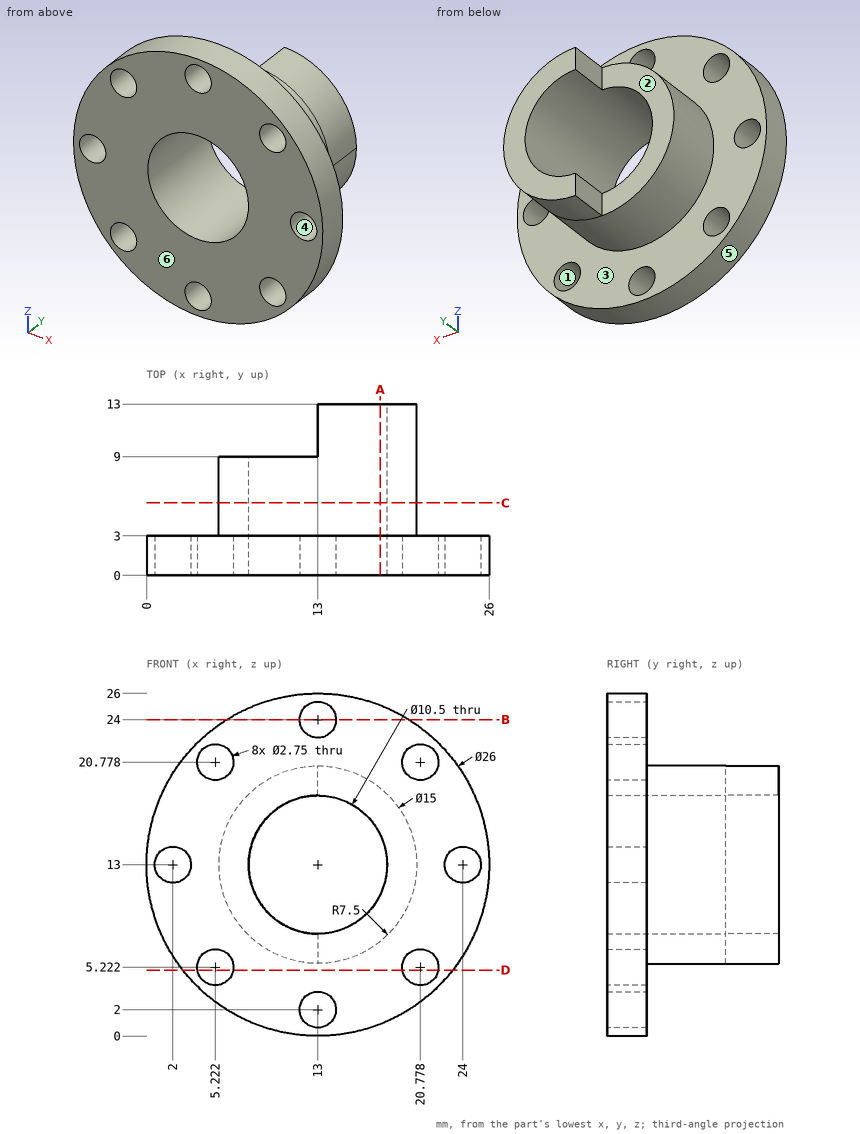
Here's the drawing with two shaded views (mm, measured from the low corner). I have some questions. A direction names the side the tool comes from. Round coordinates to 2 decimals unless told otherwise and drop trailing zeros. Order: outer loops, then holes, each group sorted by start corner. A loop starts at its lowest first (then second) coordinate and runs counter-clockwise, first axis right, second up. Notation, with made-up numbers: (-30, 52.5) -> (16, 52.5) arc R23 cw to (16, 69.5) -> close; hole circle Ø6 at (77, -13.75). An arc over 180 degrees is marked (long way). Write each question's results on one line, items separated by ' | '. Start each with the question number.
Item 1: Please list where these lines run through material, in increasing order: L1, parallel to Z at x = 19.75, y = 2.25 (1 decimal); L2, parallel to Y at x = 4, z = 19.5; L3, parallel to Z at x = 14.25, y = 2.
Item 2: If we section it at D-D, the plane z = 5: Write out the boundary of the cut face in (x, y) (1 decimal), then the cut area to 3 significant figures.
Item 3: Thinking about a two-plate mould opening in X: for the marked faces 4, 5 and 6, which applies, +X half, -X half, draft (parallel to the pull), parting line (faces both ways), or undercut?
Item 4: Which directions (+Z, -Z, +X, -X, +Y, -Y) give clear straight access to the entire face, cutting with the end or side of a thin tool? Please do the marked faces 1, 2 and 3.
Item 5: If we section it at B-B, the plane z = 24: Write out the boundary of the cut face in (x, y) (1 decimal).
Item 6: If we section it at C-C, the plane y = 5.5: Write out the boundary of the cut face in (x, z).
Item 7: If we section it at A-A, the plane x = 17.75: Write out the boundary of the cut face in (y, z), then the cut area to 3 significant figures.
Item 8: Will these pins go through, and if not, where does the flat tip stop? pin 1 (2.5 mm diameter, centred on y = 12, z = 19.5, fed in from -X); pin 2 (2 mm diameter, centred on y = 4.5, z = 16.5, fed in from -X); pin 3 (5 mm diameter, centred on x = 7, z = 20.5, fed in from +Y).
Results:
1) L1: z = 1.9 to 4.3, 6.1 to 19.9, 21.7 to 24.1 | L2: y = 0 to 3 | L3: z = 0.06 to 1.43, 2.57 to 7.9, 18.1 to 23.43, 24.57 to 25.94
2) outline: (2.8, 0) -> (3.9, 0) -> (3.9, 3) -> (2.8, 3) -> close; (6.6, 0) -> (19.4, 0) -> (19.4, 3) -> (6.6, 3) -> close; (22.1, 0) -> (23.2, 0) -> (23.2, 3) -> (22.1, 3) -> close | area: 45.2 mm2
3) face 4: undercut | face 5: parting line | face 6: draft
4) face 1: +Y, -Y | face 2: +Z, -Z, -X, +Y | face 3: +Y
5) outline: (6.1, 0) -> (11.6, 0) -> (11.6, 3) -> (6.1, 3) -> close; (14.4, 0) -> (19.9, 0) -> (19.9, 3) -> (14.4, 3) -> close
6) outline: circle Ø15 at (13, 13); hole circle Ø10.5 at (13, 13)
7) outline: (0, 0.9) -> (3, 0.9) -> (3, 7.2) -> (13, 7.2) -> (13, 10.76) -> (0, 10.76) -> close; (0, 15.24) -> (13, 15.24) -> (13, 18.8) -> (3, 18.8) -> (3, 25.1) -> (0, 25.1) -> close | area: 131 mm2
8) pin 1: stops at x = 13 | pin 2: stops at x = 5.93 | pin 3: stops at y = 9
